Could you check a few things on this model? Use its own coordinates, in mm. A direction names the side the tool comes from. Give positions to 0.01 mm unless a question says otherwise; leave off trailing zeros. Order: outer loops, then holes, each group sorted by start corner. A loop starts at its lowest first (then second) coordinate and runs counter-clockwise, first axis right, second up.
from build123d import *

# Parameters (mm, degrees)
F0_W           = 62.330626417
F0_H           = 68.3823013678
F1_DEPTH       = 12.7
F3_D           = 6.35
F3_CSINK_D     = 12.7
F3_CSINK_ANGLE = 90
F4_R           = 5.08
F5_SIZE        = 5.08
F6_W           = 42.330626417
F6_H           = 20
F7_DEPTH       = 20
F8_R           = 9.99999
F9_W           = 7.7
F9_H           = 48.0895394087
F10_DEPTH      = 50
F11_F1_R       = 2
F11_F2_R       = 2


# Not quite as in the source:
# - a fillet or chamfer is up to 0.001 mm smaller than in the source, because OpenCascade refuses the exact size


with BuildPart() as f1:
    # F0 (on Front) → F1 (new body, symmetric)
    with BuildSketch(Plane.XZ):
        with Locations((-36.5127732512, 23.8983887248)):
            Rectangle(F0_W, F0_H)
    extrude(amount=F1_DEPTH, both=True)

    # F3 (through all)
    with Locations(Plane.XZ.offset(12.7)):
        with Locations((-54.9780864596, 43.1276711741), (-25.2489887894, 27.2838656685)):
            CounterSinkHole(F3_D / 2, F3_CSINK_D / 2, counter_sink_angle=F3_CSINK_ANGLE)

    # F4
    f4_edges = [f1.edges().sort_by_distance(p)[0] for p in [
        (-36.512773, -12.7, 58.089539),
    ]]
    fillet(f4_edges, radius=F4_R)

    # F5
    f5_edges = [f1.edges().sort_by_distance(p)[0] for p in [
        (-36.512773, -12.7, -10.292762),
    ]]
    chamfer(f5_edges, length=F5_SIZE)

    # F6 (on face) → F7 (join)
    with BuildSketch(Plane(origin=(0, 12.7, 0), x_dir=(-1, 0, 0), z_dir=(0, 1, 0))):
        with Locations((36.5127732512, 9.7072380409)):
            Rectangle(F6_W, F6_H)
    extrude(amount=F7_DEPTH)

    # F8 (radius 10 in the source; OpenCascade refuses exactly that, so slightly less here)
    f8_edges = [f1.edges().sort_by_distance(p)[0] for p in [
        (-15.34746, 22.7, 19.707238),
        (-15.34746, 22.7, -0.292762),
        (-57.678086, 22.7, 19.707238),
        (-57.678086, 22.7, -0.292762),
    ]]
    fillet(f8_edges, radius=F8_R)

    # F9 (on face) → F10 (join)
    with BuildSketch(Plane.YZ.offset(-5.3474600427)):
        with Locations((3.85, 24.0447697043)):
            Rectangle(F9_W, F9_H)
    extrude(amount=F10_DEPTH)

    # F11: fillet of radius 2 on 6 edges, made by hand

    # F11_f1
    f11_f1_edges = [f1.edges().sort_by_distance(p)[0] for p in [
        (19.6525399573, 7.7, 48.0895394087),
        (19.6525399573, 0, 48.0895394087),
        (19.6525399573, 7.7, 0),
        (19.6525399573, 0, 0),
    ]]
    fillet(f11_f1_edges, radius=F11_F1_R)

    # F11_f2
    f11_f2_edges = [f1.edges().sort_by_distance(p)[0] for p in [
        (-5.3474600427, 0, 24.0447697043),
        (-5.3474600427, 7.7, 24.0447697043),
        (-5.3474600427, 7.1142135624, 0.5857864376),
        (-5.3474600427, 7.1142135624, 47.5037529711),
        (-5.3474600427, 0.5857864376, 47.5037529711),
        (-5.3474600427, 0.5857864376, 0.5857864376),
    ]]
    fillet(f11_f2_edges, radius=F11_F2_R)


solid = f1.part
Item 1: Imagine slicing it at A-A on x = 27.5. List the corners of the cut face in (y, z) for me.
Findings:
outline: (0, 2) arc R2 ccw to (2, 0) - (5.7, 0) arc R2 ccw to (7.7, 2) - (7.7, 46.09) arc R2 ccw to (5.7, 48.09) - (2, 48.09) arc R2 ccw to (0, 46.09) - close
Item 2: Imagine slicing it at D-D on z = 4. List the corners of the cut face in (x, y) for me, then the cut area to 3 significant figures.
Findings:
outline: (-67.68, -12.7) - (-5.35, -12.7) - (-5.35, -2) arc R2 cw to (-3.35, 0) - (44.65, 0) - (44.65, 7.7) - (-3.35, 7.7) arc R2 cw to (-5.35, 9.7) - (-5.35, 12.7) - (-17.14, 12.7) - (-17.14, 32.7) - (-55.89, 32.7) - (-55.89, 12.7) - (-67.68, 12.7) - close
area: 2,740 mm2
Item 3: Please list where these lines run through material, in increasing order: line 1 along Y through (x, z) = (-15.5, 51); line 2 along Y through (x, z) = (26.5, 43); line 3 along X through (y, z) = (-4.5, -6.5).
Findings:
line 1: y = -12.7 to 12.7
line 2: y = 0 to 7.7
line 3: x = -67.68 to -5.35
Item 4: We'd pull the mould along Z, two halves only. Please class faces 1 (the conical face through (-21.9, -9.7, 27.4)), 2 (the flat face through (-37, 2, 58.09)), 3 (the cylindrical face through (-54.826, 22.84, 2.714)): +Z half, -Z half, draft (parallel to the pull), parting line (faces both ways), or undercut.
Findings:
face 1: undercut
face 2: +Z half
face 3: -Z half
Item 5: For pin 1 (12 mm diameter, centred on y = 17.5, z = 18, fed in from +X); pin 2 (1.5 mm diameter, centred on x = 33, z = 38, fed in from +Y); pin 3 (4 mm diameter, centred on x = 26, y = 4, fed in from +Z), each with a flat end and sliding along its axis, tell me the tip position at first contact or that it passes through.
Findings:
pin 1: stops at x = -5.35
pin 2: stops at y = 7.7
pin 3: stops at z = 48.09
Item 6: For faces 4 (the flat face through (-36, 23, -0.293)), 5 (the flat face through (20, 4, 48.09)), 6 (the flat face through (20, 0, 24)), 7 (the flat face through (20, 7.7, 24)), which set-ups out of +Z, -Z, +X, -X, +Y, -Y let a thin tool reach every point of the face, with its end or its side?
Findings:
face 4: -Z, +X, -X, +Y
face 5: +Z, +X, +Y, -Y
face 6: +Z, -Z, +X, -Y
face 7: +Z, -Z, +X, +Y
Item 7: Imagine slicing it at B-B on y = 3.5. List the corners of the cut face in (x, z) for me (3 decimals).
Findings:
outline: (-67.678, -10.293) - (-5.347, -10.293) - (-5.347, -2) arc R2 cw to (-3.347, 0) - (44.653, 0) - (44.653, 48.09) - (-3.347, 48.09) arc R2 cw to (-5.347, 50.09) - (-5.347, 58.09) - (-67.678, 58.09) - close; hole circle Ø6.35 at (-54.978, 43.128); hole circle Ø6.35 at (-25.249, 27.284)
